```python
from build123d import *

# Parameters (mm, degrees)
BOSS_EXTRUDE1_DEPTH = 1.6
SKETCH8_3_R         = 2.5
CUT_EXTRUDE1_DEPTH  = 178.756608161
SKETCH25_R          = 2.5
CUT_EXTRUDE2_DEPTH  = 178.756608161
SKETCH16_R          = 1.6
CUT_EXTRUDE3_DEPTH  = 178.756608161
CUT_EXTRUDE6_DEPTH  = 175.275284078


with BuildPart() as part:
    # Sketch8 → Boss-Extrude1 (new body)
    with BuildSketch(Plane.XY):
        with BuildLine():
            ThreePointArc((103.534701401, 106.398987898), (103.693161759, 110.090138371), (104.446158593, 113.707139515))
            ThreePointArc((104.446158593, 113.707139515), (97.535722451, 128.659745128), (81.803110207, 123.779227301))
            ThreePointArc((81.803110207, 123.779227301), (68.396685685, 109.506582784), (50.436082024, 101.705472858))
            ThreePointArc((50.436082024, 101.705472858), (40.732585656, 91.888172428), (45.984244445, 79.122699094))
            ThreePointArc((45.984244445, 79.122699094), (60.856228216, 70.93053968), (76.976923111, 65.600382715))
            ThreePointArc((76.976923111, 65.600382715), (77.137220348, 65.563882378), (77.2977589, 65.528458486))
            ThreePointArc((77.2977589, 65.528458486), (77.354298773, 65.515492739), (77.410522602, 65.501218676))
            ThreePointArc((77.410522602, 65.501218676), (94.023303804, 63.303193357), (110.759742778, 64.144278965))
            ThreePointArc((110.759742778, 64.144278965), (121.287127646, 74.212620667), (115.130462452, 87.414620912))
            ThreePointArc((115.130462452, 87.414620912), (112.067901623, 89.481121015), (109.379631064, 92.015465685))
            ThreePointArc((109.379631064, 92.015465685), (109.377986421, 92.015505684), (109.376341775, 92.015545509))
            ThreePointArc((109.376341775, 92.015545509), (109.37615287, 92.017539878), (109.375963817, 92.019534234))
            ThreePointArc((109.375963817, 92.019534234), (105.194093866, 98.693961054), (103.534911629, 106.393514545))
            ThreePointArc((103.534911629, 106.393514545), (103.533655951, 106.395075463), (103.532400156, 106.396636288))
            ThreePointArc((103.532400156, 106.396636288), (103.533550841, 106.397812032), (103.534701401, 106.398987898))
        make_face()
    extrude(amount=BOSS_EXTRUDE1_DEPTH)

    # Sketch8<3> → Cut-Extrude1 (cut, through all)
    with BuildSketch(Plane.XY):
        with Locations((70.435309654, 103.157249982)):
            Circle(SKETCH8_3_R)
    extrude(amount=CUT_EXTRUDE1_DEPTH, mode=Mode.SUBTRACT)

    # Sketch25 → Cut-Extrude2 (cut, through all)
    with BuildSketch(Plane.XY):
        with Locations((52.996556322, 89.470524089)):
            Circle(SKETCH25_R)
        with Locations((82.496556322, 89.470524089)):
            Circle(SKETCH25_R)
        with Locations((92.45540719, 117.238694526)):
            Circle(SKETCH25_R)
        with Locations((109.001946024, 76.520067852)):
            Circle(SKETCH25_R)
    extrude(amount=CUT_EXTRUDE2_DEPTH, mode=Mode.SUBTRACT)

    # Sketch16 → Cut-Extrude3 (cut, through all)
    with BuildSketch(Plane.XY):
        with Locations((43.996556322, 89.470524089)):
            Circle(SKETCH16_R)
        with Locations((61.996556322, 89.470524089)):
            Circle(SKETCH16_R)
        with Locations((73.496556322, 89.470524089)):
            Circle(SKETCH16_R)
        with Locations((91.496556322, 89.470524089)):
            Circle(SKETCH16_R)
        with Locations((100.001946024, 76.520067852)):
            Circle(SKETCH16_R)
        with Locations((118.001946024, 76.520067852)):
            Circle(SKETCH16_R)
        with Locations((83.45540719, 117.238694526)):
            Circle(SKETCH16_R)
        with Locations((101.45540719, 117.238694526)):
            Circle(SKETCH16_R)
    extrude(amount=CUT_EXTRUDE3_DEPTH, mode=Mode.SUBTRACT)

    # Sketch23 → Cut-Extrude6 (cut, through all)
    with BuildSketch(Plane(origin=(-19.097367964, 26.776820286, 0), x_dir=(0.9781476007338056, -0.2079116908177598, 0), z_dir=(0, 0, 1))):
        Polygon((103.223291241, 65.776224437), (91.223291241, 65.776224437), (91.223291241, 59.276224437), (99.26102874, 59.276224437), (103.223291241, 60.39602146), align=None)
    extrude(amount=CUT_EXTRUDE6_DEPTH, mode=Mode.SUBTRACT)


solid = part.part
```
Source: CAD feature listing. Evaluate the final solid. Frame: model axes, mm. A direction names the side the tool comes from. Coordinates: 2 decimals unless noted, no trailing zeros. Write each loop counter-clockwise with the first axis right and the second up, starting at its lowest first coordinate (ties: lowest second). Pieces come first, ordered by that corner, then holes. Notation, with made-up numbers: (60.25, -5.5) - (101.25, -5.5) arc R9 cw to (101.25, 10.5) - close; hole circle Ø10 at (52, -34). An arc over 180 degrees is marked (long way). Answer as a JSON object with one key per item and string values.
Q1. Section query A-A, the plane y = 104.5. Output: boundary loops of the cut face in (x, z).
Ans:
{"outline": "(59.37, 0) - (68.33, 0) - (68.33, 1.6) - (59.37, 1.6) - close; (72.54, 0) - (103.69, 0) - (103.69, 1.6) - (72.54, 1.6) - close"}
Q2. First-contact query: pin 1 Ø8 at (x, y) = (112, 84) entering from -Z. Flat tip, straight axial feed; report the tip coordinate or a pass-through.
Ans:
{"pin 1": "stops at z = 0"}
Q3. Section query D-D, the plane x = 48. Output: boundary loops of the cut face in (y, z), plus the area to 3 significant figures.
Ans:
{"outline": "(77.79, 0) - (100.93, 0) - (100.93, 1.6) - (77.79, 1.6) - close", "area": "37.0 mm2"}
Q4. Material intervals for line 1 (Y direction, x = 100, z = 0.65); line 2 (Y direction, x = 101, z = 0.1); line 3 (Y direction, x = 54, z = 0.4), sorted ascending. Write a range as [from, to].
Ans:
{"line 1": "y = [63.25, 74.92], [78.12, 116.57], [117.9, 127.21]", "line 2": "y = [63.28, 75.27], [77.77, 115.7], [118.77, 126.36]", "line 3": "y = [74.27, 87.18], [91.76, 102.59]"}
Q5. Set-up query: faces 1 (the flat face through (92.344, 64.254, 0.789)), 2 (the cylindrical face through (93.789, 63.313, 0.789)). Return all of +Z, -Z, +X, -X, +Y, -Y with unobstructed straight access to the full face (end or side cutting, diameter ignored); none if empty.
Ans:
{"face 1": "+Z, -Z", "face 2": "+Z, -Z, -Y"}
Q6. Section query B-B, the plane x = 107.5. Output: boundary loops of the cut face in (y, z).
Ans:
{"outline": "(63.74, 0) - (74.52, 0) - (74.52, 1.6) - (63.74, 1.6) - close; (78.52, 0) - (94.4, 0) - (94.4, 1.6) - (78.52, 1.6) - close"}
Q7. Draft query along Y for faces 3 (the cylindrical face through (42.817, 90.552, 0.789)), 4 (the cylindrical face through (121.245, 73.999, 0.789)), 5 (the cylindrical face through (60.638, 71.026, 0.789)). Return one class per face: released by +Y, released by -Y, zero draft, split by the parting line, or undercut.
Ans:
{"face 3": "undercut", "face 4": "split by the parting line", "face 5": "released by -Y"}
Q8. Section query C-C, the plane z = 1.15. State how many separate pieces and enclosed holes the cut face has, plus the area to 3 significant figures.
Ans:
{"separate pieces": "1", "enclosed holes": "14", "area": "3,050 mm2"}
